Can you work these out from the model? Positions are in its coordinate system, mm. A direction names the side the tool comes from. Coordinates: 2 decimals unless noted, no trailing zeros. Order: outer loops, then holes, each group sorted by start corner. A loop starts at its lowest first (then second) coordinate and runs counter-clockwise, first axis right, second up. Notation, with made-up numbers: (-16.75, 54.25) -> (32.25, 54.25) arc R22 cw to (32.25, 90.25) -> close; hole circle Ø8 at (-27.75, -31). An arc over 180 degrees is marked (long way). Answer as a JSON object with one key per item and string values. Group by question number.
(1) I need wall thicknesses on line 1 (X direction, y = -56, z = 10); line 2 (Y direction, x = -59, z = 6.5); line 3 (Z direction, x = -44.5, y = -67.5). Which ranges of each line are inside material? Lowest first, please.
(2) I want a section at A-A, the plane x = 2.5. List the corners of the cut face in (y, z) for me, plus the area to 3 significant figures.
(3) For pin 1 (6 mm diameter, centred on x = 4, z = 17.5, fed in from +Y); pin 2 (1.5 mm diameter, centred on y = -75.5, z = 69.5, fed in from +X); pin 3 (12 mm diameter, centred on y = -85, z = 62, fed in from -X), each with a flat end and sliding along its axis, tell me the tip position at first contact or that it passes through.
(4) I want a section at D-D, the plane z = 16.5. State how many separate pieces and enclosed holes the cut face has, plus the area to 3 significant figures.
(5) I want a section at C-C, the plane x = -50.5. List the corners of the cut face in (y, z) for me.
(6) I want a section at B-B, the plane y = -121.5. List the corners of the cut face in (x, z) for me, plus the area to 3 significant figures.
(7) Which directions (+Z, -Z, +X, -X, +Y, -Y) give clear straight access to the entire face, cutting with the end or side of a thin tool? Please do faces 4 (the flat face through (45, -76, 80.9)), 5 (the cylindrical face through (31.681, -76.076, 12.325)), 6 (the cylindrical face through (-22.615, -112.2, 12.325)).
(8) If we mould it in two halves opening along Y, with no side actions, what happens to faces 1 (the cylindrical face through (50.68, -68.07, 52.56)), 2 (the flat face through (62, -64.09, 12)), 3 (the flat face through (-47, -32.09, 12))? For each: pulls with the +Y half, pulls with the -Y half, needs draft (parallel to the pull), parting line crosses it, or undercut.
from build123d import *

# Parameters (mm, degrees)
F1_DEPTH = 25
F3_R     = 9.716301
F4_DEPTH = 55.9


with BuildPart() as f1:
    # F0 (on Top) → F1 (new body)
    with BuildSketch(Plane.XY):
        with BuildLine():
            Line((-22.616219, -32.090175), (-72.616219, -32.090175))
            Line((-72.616219, -32.090175), (-72.616219, -112.090175))
            Line((-72.616219, -112.090175), (-72.616219, -132.090175))
            Line((-72.616219, -132.090175), (-17.616219, -132.090175))
            Line((-17.616219, -132.090175), (87.383781, -132.090175))
            Line((87.383781, -132.090175), (87.383781, -112.090175))
            Line((87.383781, -112.090175), (87.383781, -52.090175))
            Line((87.383781, -52.090175), (87.383781, -32.090175))
            Line((87.383781, -32.090175), (62.383781, -32.090175))
            Line((62.383781, -32.090175), (37.383781, -32.090175))
            Line((37.383781, -32.090175), (37.383781, -62.090175))
            ThreePointArc((37.383781, -62.090175), (31.525917, -76.23231), (17.383781, -82.090175))
            Line((17.383781, -82.090175), (-2.616219, -82.090175))
            ThreePointArc((-2.616219, -82.090175), (-16.758354, -76.23231), (-22.616219, -62.090175))
            Line((-22.616219, -62.090175), (-22.616219, -32.090175))
        make_face()
        Polygon((-40.688015, -100.090175), (-37.223914, -106.090175), (-33.759812, -112.090175), (-37.223914, -118.090175), (-40.688015, -124.090175), (-47.616219, -124.090175), (-54.544422, -124.090175), (-58.008523, -118.090175), (-61.472625, -112.090175), (-58.008523, -106.090175), (-54.544422, -100.090175), (-47.616219, -100.090175), align=None, mode=Mode.SUBTRACT)
        with BuildLine():
            ThreePointArc((-17.616219, -117.090175), (-22.616219, -112.090175), (-17.616219, -107.090175))
            Line((-17.616219, -107.090175), (32.383781, -107.090175))
            ThreePointArc((32.383781, -107.090175), (37.383781, -112.090175), (32.383781, -117.090175))
            Line((32.383781, -117.090175), (-17.616219, -117.090175))
        make_face(mode=Mode.SUBTRACT)
        Polygon((69.311985, -100.090175), (72.776086, -106.090175), (76.240188, -112.090175), (72.776086, -118.090175), (69.311985, -124.090175), (62.383781, -124.090175), (55.455578, -124.090175), (51.991477, -118.090175), (48.527375, -112.090175), (51.991477, -106.090175), (55.455578, -100.090175), (62.383781, -100.090175), align=None, mode=Mode.SUBTRACT)
        Polygon((-40.688015, -40.090175), (-37.223914, -46.090175), (-33.759812, -52.090175), (-37.223914, -58.090175), (-40.688015, -64.090175), (-47.616219, -64.090175), (-54.544422, -64.090175), (-58.008523, -58.090175), (-61.472625, -52.090175), (-58.008523, -46.090175), (-54.544422, -40.090175), (-47.616219, -40.090175), align=None, mode=Mode.SUBTRACT)
        Polygon((69.311985, -40.090175), (72.776087, -46.090175), (76.240188, -52.090175), (72.776086, -58.090175), (69.311985, -64.090175), (62.383781, -64.090175), (55.455578, -64.090175), (51.991477, -58.090175), (48.527375, -52.090175), (51.991477, -46.090175), (55.455578, -40.090175), (62.383781, -40.090175), align=None, mode=Mode.SUBTRACT)
    extrude(amount=F1_DEPTH)

    # F3 (on face) → F4 (join)
    with BuildSketch(Plane.XY.offset(25)):
        with Locations((45.454014, -76.263003)):
            Circle(F3_R)
    extrude(amount=F4_DEPTH)


solid = f1.part
Computed values:
{
 "1": {"line 1": "x = -72.62 to -59.22, -36.02 to -22.62, 37.38 to 50.78, 73.98 to 87.38", "line 2": "y = -132.09 to -116.37, -107.81 to -56.37, -47.81 to -32.09", "line 3": "z = 0 to 25"},
 "2": {"outline": "(-132.09, 0) -> (-117.09, 0) -> (-117.09, 25) -> (-132.09, 25) -> close; (-107.09, 0) -> (-82.09, 0) -> (-82.09, 25) -> (-107.09, 25) -> close", "area": "1,000 mm2"},
 "3": {"pin 1": "stops at y = -82.09", "pin 2": "stops at x = 55.17", "pin 3": "stops at x = 36.13"},
 "4": {"separate pieces": "1", "enclosed holes": "5", "area": "10,600 mm2"},
 "5": {"outline": "(-132.09, 0) -> (-124.09, 0) -> (-124.09, 25) -> (-132.09, 25) -> close; (-100.09, 0) -> (-64.09, 0) -> (-64.09, 25) -> (-100.09, 25) -> close; (-40.09, 0) -> (-32.09, 0) -> (-32.09, 25) -> (-40.09, 25) -> close"},
 "6": {"outline": "(-72.62, 0) -> (-56.04, 0) -> (-56.04, 25) -> (-72.62, 25) -> close; (-39.19, 0) -> (53.96, 0) -> (53.96, 25) -> (-39.19, 25) -> close; (70.81, 0) -> (87.38, 0) -> (87.38, 25) -> (70.81, 25) -> close", "area": "3,160 mm2"},
 "7": {"face 4": "+Z, +X, -X, +Y, -Y", "face 5": "+Z, -Z, +Y", "face 6": "+Z, -Z"},
 "8": {"face 1": "parting line crosses it", "face 2": "undercut", "face 3": "pulls with the +Y half"}
}
